Verification items for the finished model (mm, model axes). Face numbers are marked on the shaded views. A direction names the side the tool comes from. Coordinates: 2 decimals unless noted, no trailing zeros. Order: outer loops, then holes, each group sorted by start corner. A loop starts at its lowest first (then second) coordinate and runs counter-clockwise, first axis right, second up. Notation, with made-up numbers: (40, 45.25) -> (54, 45.25) arc R23 cw to (54, 54.25) -> close; hole circle Ø5 at (61.25, 79.5). An arc over 180 degrees is marked (long way). Write item = value, one per line. Start each with the question number.
1. Set-up check for the marked faces 4, 5 and 6: record each of +Z, -Z, +X, -X, +Y, -Y from which the full face is reachable in a straight line by a thin tool's end or side.
2. Release check for a two-part mould opening along Y. For the marked faces 1, 2 and 3 record: +Y half, -Y half, draft (parallel to the pull), parting line (faces both ways), or undercut.
3. Cross-section at C-C on z = 150. Record the cut outline in (x, y).
4. Cross-section at D-D on y = -177.8. Record the cut outline in (x, z), plus the area to 3 significant figures.
5. Cross-section at A-A on y = -50.8. Record the cut outline in (x, z), plus the area to 3 significant figures.
6. Cross-section at B-B on x = 133.35. Record the cut outline in (y, z), plus the area to 3 significant figures.
7. Thickness scan on line 1 along Y through (x, z) = (133.35, 5.75); line 2 along X through (y, z) = (-21.5, 24.5); line 3 along Z through (x, y) = (-105, -12). Record the ranges inside material, lowest first. Write a range as from..to.
8. Go/stop test with flat-tipped pins: P1, Ø4, axis at x = -104, y = -87.5, coming from the +Z side; P2, Ø8, axis at y = -74.5, z = 124.5, coming from the -X side; P3, Ø6, axis at x = 42.5, y = -107, coming from the -Z side; P4, Ø8, axis at x = 56.5, z = 23, coming from the +Y side. Record where each tip stops, or that it passes through.
from build123d import *

# Parameters (mm, degrees)
F1_DEPTH = 228.6
F2_W     = 190.5
F2_H     = 101.6
F3_DEPTH = 114.3
F5_DEPTH = 190.5
F8_D     = 50.8
F10_D    = 30.48


with BuildPart() as f1:
    # F0 (on Front) → F1 (new body)
    with BuildSketch(Plane.XZ):
        Polygon((-69.85, 25.4), (0, 25.4), (69.85, 25.4), (69.85, 0), (171.45, 0), (171.45, 25.4), (95.25, 25.4), (95.25, 50.8), (0, 50.8), (-95.25, 50.8), (-95.25, 25.4), (-171.45, 25.4), (-171.45, 0), (-69.85, 0), align=None)
    extrude(amount=F1_DEPTH)

    # F2 (on face) → F3 (join)
    with BuildSketch(Plane.XY.offset(50.8)):
        with Locations((0, -50.8)):
            Rectangle(F2_W, F2_H)
    extrude(amount=F3_DEPTH)

    # F4 (on face) → F5 (join)
    with BuildSketch(Plane.YZ.offset(95.25)):
        with BuildLine():
            Line((-101.6, 165.1), (0, 165.1))
            ThreePointArc((0, 165.1), (-50.8, 215.9), (-101.6, 165.1))
        make_face()
        with BuildLine():
            Line((0, 25.4), (0, 165.1))
            ThreePointArc((0, 165.1), (-50.8, 114.3), (-101.6, 165.1))
            Line((-101.6, 165.1), (-101.6, 50.8))
            Line((-101.6, 50.8), (-228.6, 50.8))
            Line((-228.6, 50.8), (-228.6, 25.4))
            Line((-228.6, 25.4), (0, 25.4))
        make_face()
    extrude(amount=-F5_DEPTH)

    # F8 (through all)
    with Locations(Plane.YZ.offset(95.25)):
        with Locations((-50.8, 165.1)):
            Hole(F8_D / 2)

    # F10 (through all)
    with Locations(Plane.XY.offset(25.4)):
        with Locations((-133.35, -50.8), (133.35, -50.8), (-133.35, -177.8), (133.35, -177.8)):
            Hole(F10_D / 2)


solid = f1.part
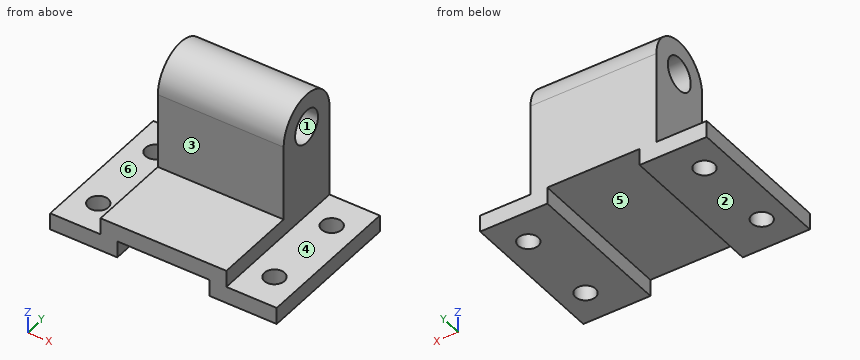
Worked out:
q1.face_4 = +Z, +X, +Y, -Y
q1.face_5 = -Z, +Y, -Y
q1.face_6 = +Z, -X, +Y, -Y
q2.face_1 = undercut
q2.face_2 = draft
q2.face_3 = -Y half
q3.outline = (-95.25, -101.6) -> (95.25, -101.6) -> (95.25, -71.22) -> (-95.25, -71.22) -> close; (-95.25, -30.38) -> (95.25, -30.38) -> (95.25, 0) -> (-95.25, 0) -> close
q4.outline = (-171.45, 0) -> (-148.59, 0) -> (-148.59, 25.4) -> (-171.45, 25.4) -> close; (-118.11, 0) -> (-69.85, 0) -> (-69.85, 25.4) -> (69.85, 25.4) -> (69.85, 0) -> (118.11, 0) -> (118.11, 25.4) -> (95.25, 25.4) -> (95.25, 50.8) -> (-95.25, 50.8) -> (-95.25, 25.4) -> (-118.11, 25.4) -> close; (148.59, 0) -> (171.45, 0) -> (171.45, 25.4) -> (148.59, 25.4) -> close
q4.area = 8,450 mm²
q5.outline = (-171.45, 0) -> (-148.59, 0) -> (-148.59, 25.4) -> (-171.45, 25.4) -> close; (-118.11, 0) -> (-69.85, 0) -> (-69.85, 25.4) -> (69.85, 25.4) -> (69.85, 0) -> (118.11, 0) -> (118.11, 25.4) -> (95.25, 25.4) -> (95.25, 139.7) -> (-95.25, 139.7) -> (-95.25, 25.4) -> (-118.11, 25.4) -> close; (-95.25, 190.5) -> (95.25, 190.5) -> (95.25, 215.9) -> (-95.25, 215.9) -> close; (148.59, 0) -> (171.45, 0) -> (171.45, 25.4) -> (148.59, 25.4) -> close
q5.area = 30,200 mm²
q6.outline = (-228.6, 0) -> (-193.04, 0) -> (-193.04, 25.4) -> (-228.6, 25.4) -> close; (-162.56, 0) -> (-66.04, 0) -> (-66.04, 25.4) -> (-162.56, 25.4) -> close; (-35.56, 0) -> (0, 0) -> (0, 25.4) -> (-35.56, 25.4) -> close
q6.area = 4,260 mm²
q7.line_1 = -228.6..-193.04, -162.56..-66.04, -35.56..0
q7.line_2 = -171.45..-69.85, 69.85..171.45
q7.line_3 = 0..25.4
q8.P1 = 25.4
q8.P2 = -95.25
q8.P3 = 25.4
q8.P4 = 0
